The listing builds one solid part. Answer for the finished solid, in the listing's coordinates (mm). Face numbers are marked on the shaded views. Give positions to 0.01 mm unless a question says otherwise; leave off trailing zeros. Order: outer loops, then holes, each group sorted by start corner. A loop starts at its lowest first (then second) coordinate and runs counter-clockwise, first axis right, second up. Notation, with made-up numbers: (2.25, -14.5) - (53.25, -14.5) arc R14 ccw to (53.25, 4.5) - close; hole circle Ø5 at (57, -25). An arc over 180 degrees is marked (long way). Answer in a Markdown table with one row per item. Add a question column.
Autodesk Inventor part; units mm, degrees
ref_plane "YZ Plane" through (0, 0, 0) normal (1, 0, 0) x (0, 1, 0)
ref_plane "XZ Plane" through (0, 0, 0) normal (0, 1, 0) x (-1, 0, 0)
ref_plane "XY Plane" through (0, 0, 0) normal (0, 0, 1) x (1, 0, 0)
sketch "Sketch1" plane through (0, 0, 0) normal (0, 1, 0) x (-1, 0, 0)
  line L0 (12.7, 12.7) -> (-12.7, 12.7)
  line L1 (-12.7, 12.7) -> (-12.7, -12.7)
  line L2 (-12.7, -12.7) -> (12.7, -12.7)
  line L3 (12.7, -12.7) -> (12.7, 12.7)
  line L4 (12.7, 12.7) -> (-12.7, -12.7) construction
  line L5 (-12.7, 12.7) -> (12.7, -12.7) construction
  line L6 (9.525, 9.525) -> (-9.525, 9.525)
  line L7 (-9.525, 9.525) -> (-9.525, -9.525)
  line L8 (-9.525, -9.525) -> (9.525, -9.525)
  line L9 (9.525, -9.525) -> (9.525, 9.525)
  line L10 (9.525, 9.525) -> (-9.525, -9.525) construction
  line L11 (-9.525, 9.525) -> (9.525, -9.525) construction
  point P0 (0, 0)
  dimension "d0" = 25.4
  dimension "d1" = 25.4
  dimension "d2" = 3.175
extrude "Extrusion1" add sketch "Sketch1" along normal mid plane 304.8
sketch "Sketch2" plane through (12.7, -152.4, -12.7) normal (1, 0, 0) x (0, 0, -1)
  line L0 (0, 0) -> (0, 304.8)
  line L1 (0, 304.8) -> (-25.4, 290.1353)
  line L2 (-25.4, 0) -> (-25.4, 304.8)
  line L3 (-25.4, 304.8) -> (0, 304.8)
  point P0 (-12.7, 152.4)
  dimension "d8" = 30
extrude "Extrusion2" cut sketch "Sketch2" against normal through all
properties part number "sideAluminumExtrusion"
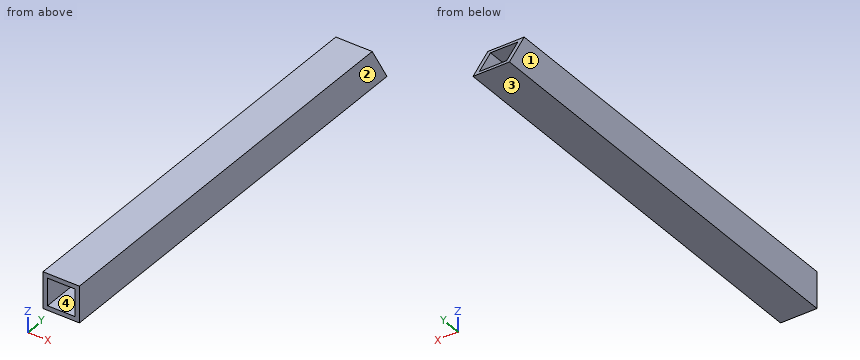
(1) Find section B-B, the plane y = 42. Write down the section's boundary in (x, z) (3 decimals).
(2) Find section C-C, the plane z = 4.5. Write down the section's boundary in (x, y) (3 decimals).
(3) The mould has two halves that part along X. Classify the marked faces 1, 2, 3 and 4: +X half, -X half, draft (parallel to the pull), parting line (faces both ways), or undercut.
(4) This flat-tipped pin is pushed along its axis until it touches: P1, Ø1, axis at x = 8.5, z = 1, coming from the +Y side. Where does it stop, or does it pass through?
(5) Straight lines are drawn through the part: line 1 (X direction, y = -129.5, z = -5) (3 decimals); line 2 (Y direction, x = 11, z = 4.25). For each, find the intervals that lie inside material, in ascending order.
(6) Find section A-A, the plane x = 1.75. Write down the section's boundary in (y, z) (3 decimals), plus the area to 3 significant figures.
Answer key:
| question | item | result |
|---|---|---|
| 1 | outline | (-12.7, -12.7) - (12.7, -12.7) - (12.7, 12.7) - (-12.7, 12.7) - close; hole (-9.525, -9.525) - (9.525, -9.525) - (9.525, 9.525) - (-9.525, 9.525) - close |
| 2 | outline | (-12.7, -152.4) - (-9.525, -152.4) - (-9.525, 142.47) - (-12.7, 142.47) - close; (9.525, -152.4) - (12.7, -152.4) - (12.7, 142.47) - (9.525, 142.47) - close |
| 3 | face 1 | -X half |
| 3 | face 2 | +X half |
| 3 | face 3 | draft |
| 3 | face 4 | undercut |
| 4 | P1 | through |
| 5 | line 1 | -12.7 to -9.525, 9.525 to 12.7 |
| 5 | line 2 | -152.4 to 142.61 |
| 6 | outline | (-152.4, -12.7) - (152.4, -12.7) - (150.567, -9.525) - (-152.4, -9.525) - close; (-152.4, 9.525) - (139.568, 9.525) - (137.735, 12.7) - (-152.4, 12.7) - close |
| 6 | area | 1,890 mm² |
